Here's the drawing with two shaded views (mm, measured from the low corner). I have some questions. A direction names the side the tool comes from. Coordinates: 2 decimals unless noted, no trailing zeros. Order: outer loops, then holes, each group sorted by start corner. A loop starts at its lowest first (then second) coordinate and runs counter-clockwise, first axis right, second up. Notation, with made-up numbers: (75.25, -12) - (133.25, -12) arc R7 ccw to (133.25, 1) - close; hole circle Ø2 at (70.5, -10.5). An arc over 180 degrees is marked (long way). One line per item, written item: value. Start each with the question number.
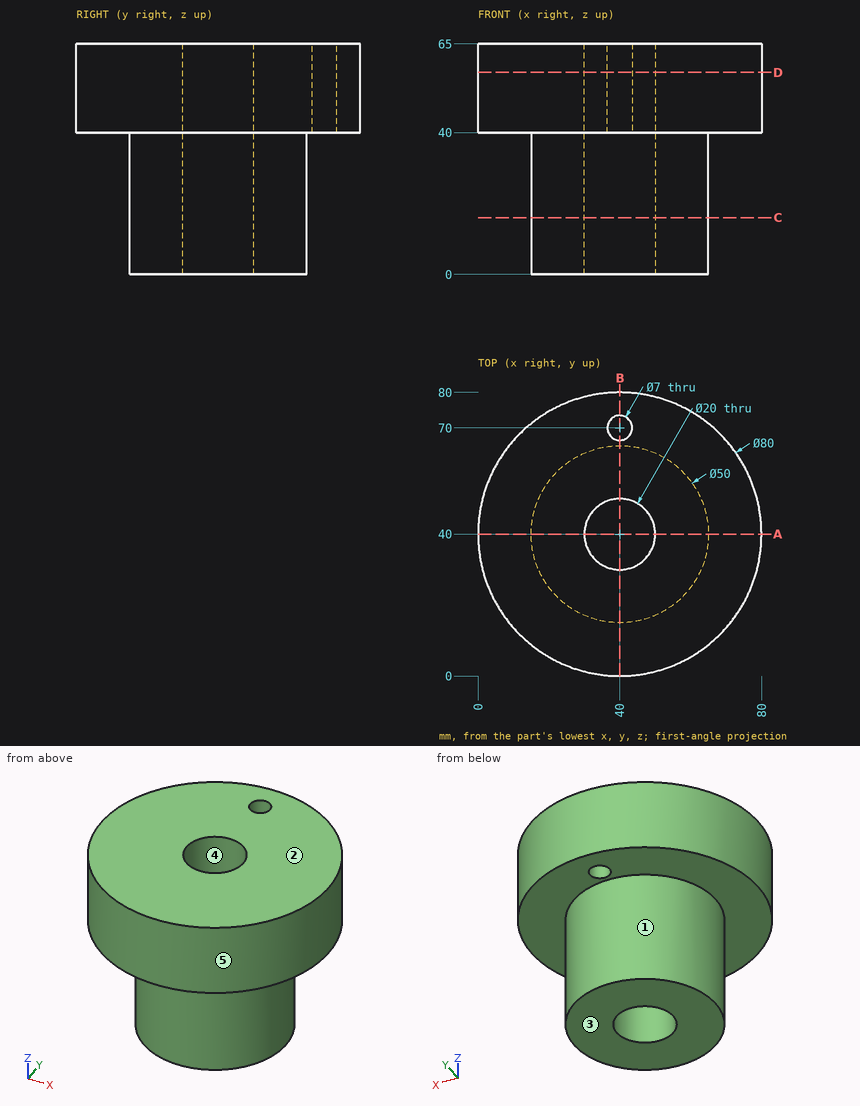
Q1. I'm going to push flat-ended pins straight in: pin 1 (12 mm diameter, centred on x = 53, z = 15.5, fed in from -Y); pin 2 (8 mm diameter, centred on x = 13.5, z = 31.5, fed in from +Y); pin 3 (3 mm diameter, centred on x = 34.5, z = 27.5, fed in from +Y). Where does each tip first touch, or does it pass through?
Q2. I want a section at B-B on x = 40. Please give me the cut outline in (y, z), then the cut area to 4 significant figures.
Q3. If I drill on L1, parallel to Y at x = 40, z = 49.5; L2, parallel to Z at x = 62.5, y = 68; L3, parallel to X at y = 32, z = 61.5, over which ranges is the centre line in solid material (lowest first)?
Q4. We'd pull the mould along X, two halves only. Please class the marked faces 3, 4 and 5: +X half, -X half, draft (parallel to the pull), parting line (faces both ways), or undercut.
Q5. I want a section at D-D on z = 57. Please give me the cut outline in (x, y).
Q6. I want a section at A-A on y = 40. Please give me the cut outline in (x, z).
Q7. Which directions (+Z, -Z, +X, -X, +Y, -Y) give clear straight access to the entire face, cutting with the end or side of a thin tool? Please do the marked faces 1 and 2.
Q8. I want a section at C-C on z = 16. Please give me the cut outline in (x, y).
Values follow:
1. pin 1: stops at y = 16
1. pin 2: stops at y = 50.9
1. pin 3: stops at y = 64.68
2. outline: (0, 40) - (15, 40) - (15, 0) - (30, 0) - (30, 65) - (0, 65) - close; (50, 0) - (65, 0) - (65, 40) - (66.5, 40) - (66.5, 65) - (50, 65) - close; (73.5, 40) - (80, 40) - (80, 65) - (73.5, 65) - close
2. area: 2,525 mm^2
3. L1: y = 0 to 30, 50 to 66.5, 73.5 to 80
3. L2: z = 40 to 65
3. L3: x = 0.81 to 34, 46 to 79.19
4. face 3: draft
4. face 4: undercut
4. face 5: parting line
5. outline: circle Ø80 at (40, 40); hole circle Ø20 at (40, 40); hole circle Ø7 at (40, 70)
6. outline: (0, 40) - (15, 40) - (15, 0) - (30, 0) - (30, 65) - (0, 65) - close; (50, 0) - (65, 0) - (65, 40) - (80, 40) - (80, 65) - (50, 65) - close
7. face 1: -Z
7. face 2: +Z, +X, -X, +Y, -Y
8. outline: circle Ø50 at (40, 40); hole circle Ø20 at (40, 40)
